The figure shows three views and two pictorial views of one solid part (mm, origin at its lowest corner). Answer the questions. A direction names the side the tool comes from. Give positions to 0.01 mm unless a question says otherwise; leave off trailing zeros. Order: outer loops, then holes, each group sorted by start corner. A loop starts at its lowest first (then second) coordinate and runs counter-clockwise, first axis right, second up. Notation, with made-up numbers: (41.25, 52.25) - (53.25, 52.25) arc R28 ccw to (53.25, 89.25) - close; hole circle Ø2 at (-28, 47). An arc over 180 degrees is marked (long way). Answer as a JSON object with one key per item and string values. Group by question number.
Q1. A cutting plane is placed at D-D, the plane y = 68.5. Give the vertices of the cut face in (x, z).
Q2. The mould has two halves that part along X. Classify the marked faces 3, 4 and 5: released by +X, released by -X, zero draft, split by the parting line, or undercut.
Q3. A cutting plane is placed at A-A, the plane x = 13. Give the vertices of the cut face in (y, z) (3 decimals), and give its area (3 significant figures).
Q4. For the marked faces 1 and 2, determine the directions among +Z, -Z, +X, -X, +Y, -Y from which every point of the face is accessible in a straight line to the end or side of a thin tool.
Q5. Consider line 1 (Y direction, x = 11.25, z = 8.25); line 2 (Y direction, x = 21.25, z = 7.5); line 3 (Z direction, x = 10.25, y = 5.5). Determine where each line is inside the solid, lowest interval first.
Q6. Given pin 1 (5.5 mm diameter, centred on y = 28, z = 7, fed in from -X); pin 2 (5 mm diameter, centred on y = 53, z = 7, fed in from -X); pin 3 (3 mm diameter, centred on y = 37.5, z = 1, fed in from +X), each flat-ended and moving along its own axis, determine where each tip first touches the part or whether it passes through.
Q7. A cutting plane is placed at C-C, the plane z = 3.5. Give the vertices of the cut face in (x, y) (1 decimal), and give its area (3 significant figures).
Q8. A cutting plane is placed at B-B, the plane y = 10. Give the vertices of the cut face in (x, z).
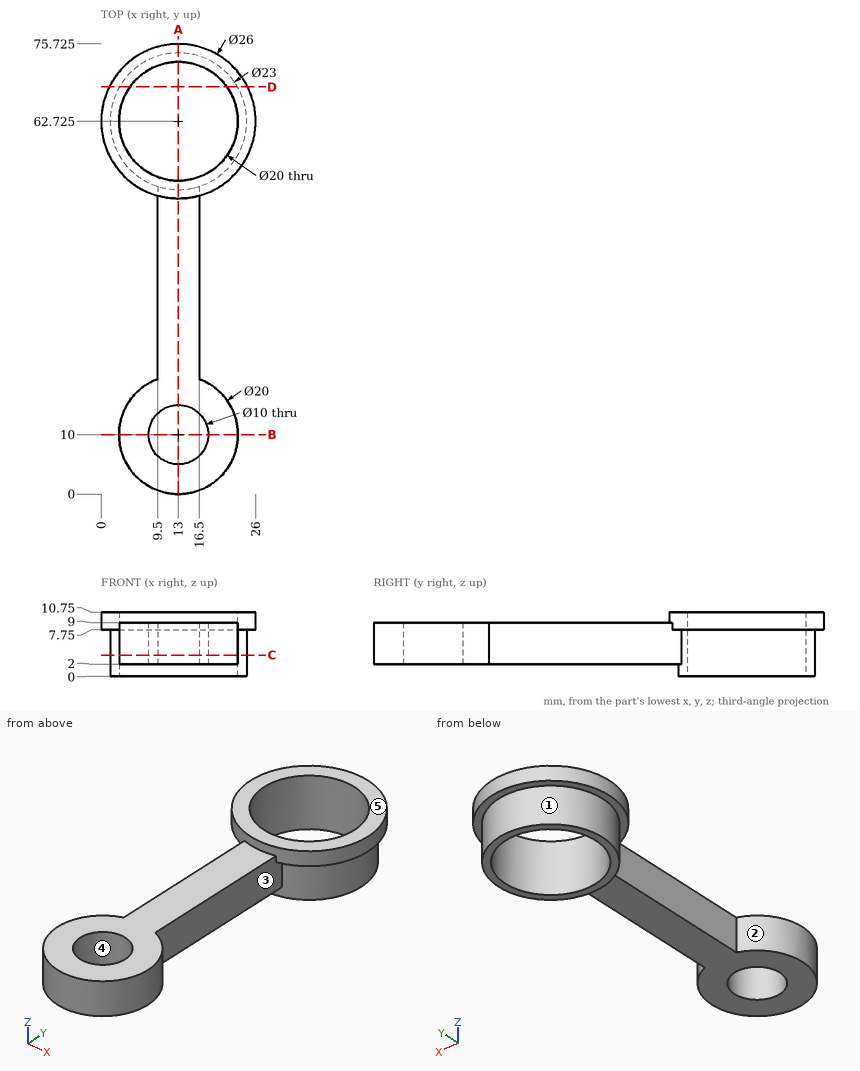
Reply:
{
 "1": {"outline": "(1.35, 7.75) - (3.06, 7.75) - (3.06, 0) - (4.84, 0) - (4.84, 10.75) - (1.35, 10.75) - close; (21.16, 0) - (22.94, 0) - (22.94, 7.75) - (24.65, 7.75) - (24.65, 10.75) - (21.16, 10.75) - close"},
 "2": {"face 3": "released by +X", "face 4": "undercut", "face 5": "zero draft"},
 "3": {"outline": "(0, 2) - (5, 2) - (5, 9) - (0, 9) - close; (15, 2) - (51.225, 2) - (51.225, 0) - (52.725, 0) - (52.725, 10.75) - (49.725, 10.75) - (49.725, 9) - (15, 9) - close; (72.725, 0) - (74.225, 0) - (74.225, 7.75) - (75.725, 7.75) - (75.725, 10.75) - (72.725, 10.75) - close", "area": "328 mm^2"},
 "4": {"face 1": "-Z", "face 2": "+Z, -Z"},
 "5": {"line 1": "y = 0.15 to 5.32, 14.68 to 52.88, 72.57 to 75.61", "line 2": "y = 4.35 to 15.65, 54.71 to 57.07, 68.38 to 70.74", "line 3": "z = 2 to 9"},
 "6": {"pin 1": "stops at x = 9.5", "pin 2": "stops at x = 2.27", "pin 3": "stops at x = 16.5"},
 "7": {"outline": "(9.5, 19.4) arc R10 ccw (long way) to (16.5, 19.4) - (16.5, 51.8) arc R11.5 ccw (long way) to (9.5, 51.8) - close; hole circle Ø20 at (13, 62.7); hole circle Ø10 at (13, 10)", "area": "558 mm^2"},
 "8": {"outline": "(3, 2) - (8, 2) - (8, 9) - (3, 9) - close; (18, 2) - (23, 2) - (23, 9) - (18, 9) - close"}
}
